Check sheet for the modelled part. Datum: model origin and axes. Units: mm. A direction names the side the tool comes from. Give positions to 0.01 mm unless a question says otherwise; leave off trailing zeros. Order: outer loops, then holes, each group sorted by start corner. A loop starts at its lowest first (then second) coordinate and runs counter-clockwise, first axis right, second up. Notation, with made-up numbers: (42, 49) -> (87, 49) arc R11 cw to (87, 66) -> close; hole circle Ø10 at (43.25, -26.75). An arc over 180 degrees is marked (long way). Answer in a Markdown table with one row per item. Add a question column.
(1) Thickness scan on L1, parallel to X at y = 3.7, z = -10.25 (3 decimals); L2, parallel to X at y = 2.7, z = 9.75; L3, parallel to Z at x = -6, y = 2.2. Record the ranges inside material, lowest first. Write a range as [from, to].
(2) Cross-section at B-B (y = 3.45). State how many separate pieces and enclosed holes the cut face has, then the cut area to 3 significant figures.
(3) Set-up check for faces 4 (the face through (2, 2, 12.5)), 5 (the face through (20.56, 1.97, 10.61)), 6 (the face through (14, 4.5, 0.1)): record each of +Z, -Z, +X, -X, +Y, -Y from which the full face is reachable in a straight line by a thin tool's end or side.
(4) Release check for a two-part mould opening along Z. For faces 1 (the face through (13.54, 4.49, -5.27)), 2 (the face through (-24.5, 3, 0)), 3 (the face through (-23.56, 2.46, -11.61)) record: released by +Z, released by -Z, zero draft, split by the parting line, or undercut.
(5) Cross-section at A-A (z = -0.5). Record the cut outline in (x, y) (3 decimals), then the cut area to 4 significant figures.
(6) Go/stop test with flat-tipped pins: pin 1 (3 mm diameter, centred on x = -19, z = 6.5, fed in from -Y); pin 2 (3 mm diameter, centred on x = -1, z = -3.5, fed in from -Y); pin 3 (6 mm diameter, centred on x = 15, z = -7, fed in from -Y); pin 4 (1.1 mm diameter, centred on y = 4.5, z = -2, fed in from +X). Record where each tip stops, or that it passes through.
```python
from build123d import *

# Parameters (mm, degrees)
BOSS_EXTRUDE1_DEPTH = 5
SKETCH2_W           = 28
SKETCH2_H           = 11.5
CUT_EXTRUDE1_DEPTH  = 27.220221204253797
SHELL1_T            = -1
FILLET1_R           = 1.6
FILLET2_R           = 3.125
BOSS_EXTRUDE2_DEPTH = 5
FILLET3_R           = 3.125
FILLET4_R           = 3.125
BOSS_EXTRUDE3_START = -5
BOSS_EXTRUDE3_DEPTH = 5
FILLET5_R           = 3.125
SKETCH7_R           = 1.0250000000000001
CUT_EXTRUDE2_DEPTH  = 31.730939361252858


with BuildPart() as part:
    # Sketch1 → Boss-Extrude1 (new body)
    with BuildSketch(Plane(origin=(0, 0, 0), x_dir=(1, 0, 0), z_dir=(0, 1, 0))):
        Polygon((-22.500000000000007, 12.500000000000004), (22.499999999999996, 12.500000000000004), (22.499999999999996, -12.499999999999996), (-22.500000000000004, -12.499999999999996), align=None)
    extrude(amount=BOSS_EXTRUDE1_DEPTH)

    # Sketch2 → Cut-Extrude1 (cut, through all)
    with BuildSketch(Plane(origin=(0, 5, 0), x_dir=(1, 0, 0), z_dir=(0, 1, 0))):
        Rectangle(SKETCH2_W, SKETCH2_H)
    extrude(amount=-CUT_EXTRUDE1_DEPTH, mode=Mode.SUBTRACT)

    # Shell1
    shell1_openings = [part.faces().sort_by_distance(p)[0] for p in [
        (14, 2.5, 0),
        (0, 2.5, 5.75),
        (-14, 2.5, 0),
        (0, 2.5, -5.75),
        (0, 0, -11.985218493),
    ]]
    offset(amount=SHELL1_T, openings=shell1_openings, kind=Kind.INTERSECTION)

    # Fillet1
    fillet1_edges = [part.edges().sort_by_distance(p)[0] for p in [
        (14.000000000000002, 4.5, -5.750000000000001),
        (14.000000000000002, 4.5, 5.749999999999999),
        (-13.999999999999998, 4.5, 5.749999999999999),
        (-13.999999999999998, 4.5, -5.750000000000001),
    ]]
    fillet(fillet1_edges, radius=FILLET1_R)

    # Fillet2
    fillet2_edges = [part.edges().sort_by_distance(p)[0] for p in [
        (21.499999999999996, 2, 11.499999999999996),
        (21.499999999999993, 2, -11.500000000000004),
        (-21.500000000000007, 2, -11.500000000000004),
        (-21.500000000000004, 2, 11.499999999999996),
    ]]
    fillet(fillet2_edges, radius=FILLET2_R)

    # Sketch4 → Boss-Extrude2 (add)
    with BuildSketch(Plane.XZ):
        with BuildLine():
            Line((22.499999999999996, 12.499999999999996), (22.499999999999996, -12.500000000000004))
            Line((22.499999999999996, -12.500000000000004), (37, -12.5))
            ThreePointArc((37, -12.500000000000002), (24.5, 6.814e-14), (37.000000000000135, 12.500000000000002))
            Line((37.000000000000135, 12.500000000000002), (22.499999999999996, 12.499999999999996))
        make_face()
    extrude(amount=-BOSS_EXTRUDE2_DEPTH)

    # Fillet3
    fillet3_edges = [part.edges().sort_by_distance(p)[0] for p in [
        (37, 2.5, -12.5),
    ]]
    fillet(fillet3_edges, radius=FILLET3_R)
    fillet3_2_edges = [part.edges().sort_by_distance(p)[0] for p in [
        (37.000000000000135, 2.5, 12.5),
    ]]
    fillet(fillet3_2_edges, radius=FILLET3_R)

    # Fillet4
    fillet4_edges = [part.edges().sort_by_distance(p)[0] for p in [
        (-22.500000000000004, 2.5, 12.499999999999996),
        (-22.500000000000007, 2.5, -12.500000000000004),
    ]]
    fillet(fillet4_edges, radius=FILLET4_R)

    # Sketch6 → Boss-Extrude3 (add)
    with BuildSketch(Plane.XZ.offset(BOSS_EXTRUDE3_START)):
        with BuildLine():
            ThreePointArc((-21.500000000000004, -8.375000000000004), (-20.584708691207968, -10.584708691207965), (-18.375000000000007, -11.500000000000004))
            Line((-18.375000000000004, -11.500000000000004), (-18.375000000000004, 11.499999999999996))
            ThreePointArc((-18.375000000000004, 11.499999999999996), (-20.58470869120796, 10.584708691207954), (-21.5, 8.374999999999996))
            Line((-21.5, 8.374999999999996), (-21.500000000000004, -8.375000000000004))
        make_face()
        Polygon((-24.5, -12.500000000000004), (-22.500000000000007, -12.500000000000004), (-22.500000000000007, -9.375000000000005), (-22.500000000000004, 9.374999999999996), (-22.500000000000004, 12.499999999999996), (-24.5, 12.499999999999991), align=None)
        with BuildLine():
            Line((-22.500000000000004, 9.374999999999996), (-22.500000000000007, -9.375000000000005))
            ThreePointArc((-22.500000000000007, -9.375000000000005), (-21.584708691207968, -11.584708691207966), (-19.375000000000007, -12.500000000000002))
            Line((-19.375000000000007, -12.500000000000004), (-18.375000000000004, -12.500000000000004))
            Line((-18.375000000000004, -12.500000000000004), (-18.375000000000004, -11.500000000000004))
            ThreePointArc((-18.375000000000007, -11.500000000000004), (-20.584708691207968, -10.584708691207965), (-21.500000000000004, -8.375000000000004))
            Line((-21.500000000000004, -8.375000000000004), (-21.5, 8.374999999999996))
            ThreePointArc((-21.5, 8.374999999999996), (-20.58470869120796, 10.584708691207954), (-18.375000000000004, 11.499999999999996))
            Line((-18.375000000000004, 11.499999999999996), (-18.375000000000004, 12.499999999999996))
            Line((-18.375000000000004, 12.499999999999996), (-19.375000000000004, 12.499999999999996))
            ThreePointArc((-19.375000000000004, 12.499999999999996), (-21.584708691207965, 11.584708691207958), (-22.500000000000004, 9.374999999999998))
        make_face()
        with BuildLine():
            Line((-22.500000000000007, -9.375000000000005), (-22.500000000000007, -12.500000000000004))
            Line((-22.500000000000007, -12.500000000000004), (-19.375000000000007, -12.500000000000004))
            ThreePointArc((-19.375000000000007, -12.500000000000002), (-21.584708691207968, -11.584708691207966), (-22.500000000000007, -9.375000000000005))
        make_face()
        with BuildLine():
            Line((-22.500000000000004, 12.499999999999996), (-22.500000000000004, 9.374999999999996))
            ThreePointArc((-22.500000000000004, 9.374999999999998), (-21.584708691207965, 11.584708691207958), (-19.375000000000004, 12.499999999999996))
            Line((-19.375000000000004, 12.499999999999996), (-22.500000000000004, 12.499999999999996))
        make_face()
    extrude(amount=BOSS_EXTRUDE3_DEPTH)

    # Fillet5
    fillet5_edges = [part.edges().sort_by_distance(p)[0] for p in [
        (-24.5, 2.5, 12.49999999999999),
        (-24.5, 2.5, -12.500000000000004),
        (-18.375000000000004, 2, 11.499999999999996),
        (-18.375000000000007, 2, -11.500000000000004),
    ]]
    fillet(fillet5_edges, radius=FILLET5_R)

    # Sketch7 → Cut-Extrude2 (cut, through all)
    with BuildSketch(Plane(origin=(0, 0, 0), x_dir=(-1, 0, 0), z_dir=(0, -1, 0))):
        with Locations(Location((-24.499999999999996, 9.375000000000005, 0), (0, 0, 90))):
            Circle(SKETCH7_R)
        with Locations(Location((-24.499999999999996, -9.375000000000005, 0), (0, 0, 90))):
            Circle(SKETCH7_R)
        with Locations(Location((21.375, -9.375000000000005, 0), (0, 0, 90))):
            Circle(SKETCH7_R)
        with Locations(Location((21.375, 9.375000000000005, 0), (0, 0, 90))):
            Circle(SKETCH7_R)
    extrude(amount=-CUT_EXTRUDE2_DEPTH, mode=Mode.SUBTRACT)


solid = part.part
```
Answer below:
| question | item | result |
|---|---|---|
| 1 | L1 | x = [-24.375, -21.909], [-20.841, -17.75], [20.875, 23.966], [25.034, 27.5] |
| 1 | L2 | x = [-24.48, -22.33], [-20.42, -18.06], [21.18, 23.55], [25.45, 27.6] |
| 1 | L3 | z = [-12.5, -11.5], [11.5, 12.5] |
| 2 | separate pieces | 1 |
| 2 | enclosed holes | 5 |
| 2 | area | 337 mm² |
| 3 | face 4 | +Z, +X, -X, +Y, -Y |
| 3 | face 5 | -Y |
| 3 | face 6 | +Y, -Y |
| 4 | face 1 | undercut |
| 4 | face 2 | zero draft |
| 4 | face 3 | released by -Z |
| 5 | outline | (-24.5, 0) -> (-18.375, 0) -> (-18.375, 4) -> (-14, 4) -> (-14, 5) -> (-24.5, 5) -> close; (14, 4) -> (21.5, 4) -> (21.5, 0) -> (24.51, 0) -> (24.51, 5) -> (14, 5) -> close |
| 5 | area | 57.55 mm² |
| 6 | pin 1 | stops at y = 0 |
| 6 | pin 2 | passes through |
| 6 | pin 3 | stops at y = 4 |
| 6 | pin 4 | stops at x = 24.76 |
